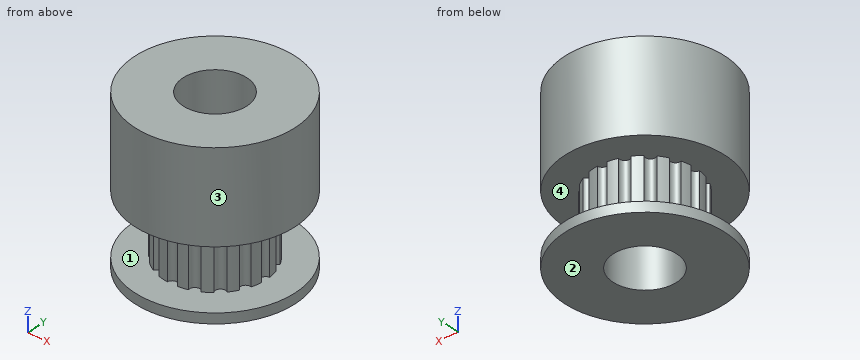
```python
from build123d import *

# Parameters (mm, degrees)
SKETCH1_R           = 8
SKETCH1_R_2         = 3.175
BOSS_EXTRUDE1_DEPTH = 1
BOSS_EXTRUDE2_DEPTH = 6
SKETCH3_R           = 8
BOSS_EXTRUDE3_DEPTH = 9
SKETCH1_3_R         = 3.175
CUT_EXTRUDE1_DEPTH  = 20.595917942


with BuildPart() as part:
    # Sketch1 → Boss-Extrude1 (new body)
    # profile 1 of 2: a face of its own
    with BuildSketch(Plane.XY):
        Circle(SKETCH1_R)
        Circle(SKETCH1_R_2, mode=Mode.SUBTRACT)
    # profile 2 of 2: a face of its own
    with BuildSketch(Plane.XY):
        Circle(SKETCH1_R_2)
    extrude(amount=BOSS_EXTRUDE1_DEPTH)

    # Sketch2 → Boss-Extrude2 (add)
    with BuildSketch(Plane.XY.offset(1)):
        with BuildLine():
            ThreePointArc((-0.499397244, 5.068414486), (-0.993586851, 4.995098416), (-1.47821536, 4.873715458))
            ThreePointArc((-1.47821536, 4.873715458), (-1.757649001, 4.243340055), (-2.400981144, 4.491493355))
            ThreePointArc((-2.400981144, 4.491493355), (-2.829495962, 4.234639963), (-3.230783076, 3.937037431))
            ThreePointArc((-3.230783076, 3.937037431), (-3.247711874, 3.247711874), (-3.937037431, 3.230783076))
            ThreePointArc((-3.937037431, 3.230783076), (-4.234639963, 2.829495962), (-4.491493355, 2.400981144))
            ThreePointArc((-4.491493355, 2.400981144), (-4.243340055, 1.757649001), (-4.873715458, 1.47821536))
            ThreePointArc((-4.873715458, 1.47821536), (-4.995098416, 0.993586851), (-5.068414486, 0.499397244))
            ThreePointArc((-5.068414486, 0.499397244), (-4.592958179, 0), (-5.068414486, -0.499397244))
            ThreePointArc((-5.068414486, -0.499397244), (-4.995098416, -0.993586851), (-4.873715458, -1.47821536))
            ThreePointArc((-4.873715458, -1.47821536), (-4.243340055, -1.757649001), (-4.491493355, -2.400981144))
            ThreePointArc((-4.491493355, -2.400981144), (-4.234639963, -2.829495962), (-3.937037431, -3.230783076))
            ThreePointArc((-3.937037431, -3.230783076), (-3.247711874, -3.247711874), (-3.230783076, -3.937037431))
            ThreePointArc((-3.230783076, -3.937037431), (-2.829495962, -4.234639963), (-2.400981144, -4.491493355))
            ThreePointArc((-2.400981144, -4.491493355), (-1.757649001, -4.243340055), (-1.47821536, -4.873715458))
            ThreePointArc((-1.47821536, -4.873715458), (-0.993586851, -4.995098416), (-0.499397244, -5.068414486))
            ThreePointArc((-0.499397244, -5.068414486), (0, -4.592958179), (0.499397244, -5.068414486))
            ThreePointArc((0.499397244, -5.068414486), (0.993586851, -4.995098416), (1.47821536, -4.873715458))
            ThreePointArc((1.47821536, -4.873715458), (1.757649001, -4.243340055), (2.400981144, -4.491493355))
            ThreePointArc((2.400981144, -4.491493355), (2.829495962, -4.234639963), (3.230783076, -3.937037431))
            ThreePointArc((3.230783076, -3.937037431), (3.247711874, -3.247711874), (3.937037431, -3.230783076))
            ThreePointArc((3.937037431, -3.230783076), (4.234639963, -2.829495962), (4.491493355, -2.400981144))
            ThreePointArc((4.491493355, -2.400981144), (4.243340055, -1.757649001), (4.873715458, -1.47821536))
            ThreePointArc((4.873715458, -1.47821536), (4.995098416, -0.993586851), (5.068414486, -0.499397244))
            ThreePointArc((5.068414486, -0.499397244), (4.592958179, 0), (5.068414486, 0.499397244))
            ThreePointArc((5.068414486, 0.499397244), (4.995098416, 0.993586851), (4.873715458, 1.47821536))
            ThreePointArc((4.873715458, 1.47821536), (4.243340055, 1.757649001), (4.491493355, 2.400981144))
            ThreePointArc((4.491493355, 2.400981144), (4.234639963, 2.829495962), (3.937037431, 3.230783076))
            ThreePointArc((3.937037431, 3.230783076), (3.247711874, 3.247711874), (3.230783076, 3.937037431))
            ThreePointArc((3.230783076, 3.937037431), (2.829495962, 4.234639963), (2.400981144, 4.491493355))
            ThreePointArc((2.400981144, 4.491493355), (1.757649001, 4.243340055), (1.47821536, 4.873715458))
            ThreePointArc((1.47821536, 4.873715458), (0.993586851, 4.995098416), (0.499397244, 5.068414486))
            ThreePointArc((0.499397244, 5.068414486), (0, 4.592958179), (-0.499397244, 5.068414486))
        make_face()
    extrude(amount=BOSS_EXTRUDE2_DEPTH)

    # Sketch3 → Boss-Extrude3 (add)
    with BuildSketch(Plane.XY.offset(7)):
        Circle(SKETCH3_R)
    extrude(amount=BOSS_EXTRUDE3_DEPTH)

    # Sketch1_3 → Cut-Extrude1 (cut, through all)
    with BuildSketch(Plane.XY):
        Circle(SKETCH1_3_R)
    extrude(amount=CUT_EXTRUDE1_DEPTH, mode=Mode.SUBTRACT)


solid = part.part
```
The model under review builds one solid part; all positions refer to its coordinate system, in mm. Face numbers are marked on the shaded views. Round coordinates to 2 decimals unless told otherwise and drop trailing zeros. Write each loop counter-clockwise with the first axis right and the second up, starting at its lowest first coordinate (ties: lowest second). Pieces come first, ordered by that corner, then holes. Notation, with made-up numbers: (83, 73) - (138, 73) arc R10 ccw to (138, 78) - close; hole circle Ø6 at (17.5, 35.25). An arc over 180 degrees is marked (long way). One line per question, with ' | ' between items.
Item 1: To check wall thickness, follow probe 1 along Y at (x, z) = (0, 12) (3 decimals); probe 2 along Z at (x, y) = (4.5, 3.5); probe 3 along X at (y, z) = (-1, 8). State the ranges of each line that lie inside material, in increasing order.
Resolved:
probe 1: y = -8 to -3.175, 3.175 to 8 | probe 2: z = 0 to 1, 7 to 16 | probe 3: x = -7.94 to -3.01, 3.01 to 7.94
Item 2: The part is to be moulded in two halves that separate along Z. For the marked faces 1, 2, 3 and 4, say which applies: pulls with the +Z half, pulls with the -Z half, needs draft (parallel to the pull), parting line crosses it, or undercut.
Resolved:
face 1: undercut | face 2: pulls with the -Z half | face 3: needs draft | face 4: undercut
Item 3: For P1, Ø1.5, axis at x = 3, z = 13, coming from the -Y side; P2, Ø4, axis at y = 2.5, z = 12, coming from the +X side; P3, Ø1.5, axis at x = -6, y = 5.5, coming from the +Z side, all flat-tipped, find the tip position at first contact; note any pin that passes through.
Resolved:
P1: stops at y = -7.68 | P2: stops at x = 7.98 | P3: stops at z = 16
Item 4: Add section B-B, the plane y = 0. Give the boundary of the cut face in (x, z) (3 decimals).
Resolved:
outline: (-8, 0) - (-3.175, 0) - (-3.175, 16) - (-8, 16) - (-8, 7) - (-4.593, 7) - (-4.593, 1) - (-8, 1) - close; (3.175, 0) - (8, 0) - (8, 1) - (4.593, 1) - (4.593, 7) - (8, 7) - (8, 16) - (3.175, 16) - close
Item 5: Add section D-D, the plane y = -6.5. Give the boundary of the cut face in (x, z).
Resolved:
outline: (-4.66, 0) - (4.66, 0) - (4.66, 1) - (-4.66, 1) - close; (-4.66, 7) - (4.66, 7) - (4.66, 16) - (-4.66, 16) - close
